from build123d import *

# Parameters (mm, degrees)
SKETCH1_R           = 2.032
BOSS_EXTRUDE1_DEPTH = 1.5875
FILLET1_R           = 6.35
FILLET2_R           = 3.175


with BuildPart() as part:
    # Sketch1 → Boss-Extrude1 (new body)
    with BuildSketch(Plane.XY):
        Polygon((9.525, -4.392368296), (9.525, 7.671504431), (3.175, 50.8), (-9.525, 50.8), (-15.875, 7.671504431), (-22.225, 1.957631704), (-22.225, -4.392368296), align=None)
        Circle(SKETCH1_R, mode=Mode.SUBTRACT)
        with Locations((-12.7, 0)):
            Circle(SKETCH1_R, mode=Mode.SUBTRACT)
    extrude(amount=BOSS_EXTRUDE1_DEPTH)

    # Fillet1
    fillet1_edges = [part.edges().sort_by_distance(p)[0] for p in [
        (-9.525, 50.8, 0.79375),
        (3.175, 50.8, 0.79375),
    ]]
    fillet(fillet1_edges, radius=FILLET1_R)

    # Fillet2
    fillet2_edges = [part.edges().sort_by_distance(p)[0] for p in [
        (-22.225, -4.392368296, 0.79375),
        (-22.225, 1.957631704, 0.79375),
        (-15.875, 7.671504431, 0.79375),
        (9.525, 7.671504431, 0.79375),
        (9.525, -4.392368296, 0.79375),
    ]]
    fillet(fillet2_edges, radius=FILLET2_R)


solid = part.part
Geometry check sheet. Reference: the model listing, model coordinates, mm. Round coordinates to 2 decimals unless told otherwise and drop trailing zeros. Order: outer loops, then holes, each group sorted by start corner. A loop starts at its lowest first (then second) coordinate and runs counter-clockwise, first axis right, second up. Notation, with made-up numbers: M 12.5,78 L 37.5,78 A21 ccw 37.5,98 Z; hole C 25.5,-21 d2. An arc over 180 degrees is marked long. Answer in a Markdown table with one row per item.
(1) Go/stop test with flat-tipped pins: P1, Ø6.5, axis at x = -12.7, y = 0, coming from the -Z side; P2, Ø1.5, axis at x = -16, y = 23, coming from the +Z side. Record where each tip stops, or that it passes through.
Responses:
| item | result |
|---|---|
| P1 | stops at z = 0 |
| P2 | passes through |
(2) Scan lines: probe 1 along Y at (x, z) = (0, 1.1); probe 2 along X at (y, z) = (19.5, 1.35); probe 3 along Y at (x, z) = (-5, 1.2). Record each from-to range of solid material in increasing order. Write a range as from..to.
Responses:
| item | result |
|---|---|
| probe 1 | y = -4.39..-2.03, 2.03..50.37 |
| probe 2 | x = -14.13..7.78 |
| probe 3 | y = -4.39..50.73 |
(3) Draft check along Y on faces 1 (the face through (-14.73, 0.09, 0.78)), 2 (the face through (-0.44, -1.984, 0.783)), 3 (the face through (-21.27, -3.49, 0.8)), 4 (the face through (-3, 50.8, 1)). Enter one of: released by +Y, released by -Y, zero draft, split by the parting line, or undercut.
Responses:
| item | result |
|---|---|
| face 1 | undercut |
| face 2 | undercut |
| face 3 | released by -Y |
| face 4 | released by +Y |
(4) Sectioned sample at D-D, the plane x = -12.7. Record the cut outline in (y, z).
Responses:
| item | result |
|---|---|
| outline | M -4.39,0 L -2.03,0 L -2.03,1.59 L -4.39,1.59 Z; M 2.03,0 L 29.24,0 L 29.24,1.59 L 2.03,1.59 Z |
(5) Sectioned sample at C-C, the plane x = -1. Record the cut outline in (y, z).
Responses:
| item | result |
|---|---|
| outline | M -4.39,0 L -1.77,0 L -1.77,1.59 L -4.39,1.59 Z; M 1.77,0 L 50.66,0 L 50.66,1.59 L 1.77,1.59 Z |
(6) Sectioned sample at B-B, the plane y = 0. Record the cut outline in (x, z) (1 decimal), and give its area (3 significant figures).
Responses:
| item | result |
|---|---|
| outline | M -22.2,0 L -14.7,0 L -14.7,1.6 L -22.2,1.6 Z; M -10.7,0 L -2,0 L -2,1.6 L -10.7,1.6 Z; M 2,0 L 9.5,0 L 9.5,1.6 L 2,1.6 Z |
| area | 37.5 mm² |
(7) Sectioned sample at A-A, the plane z = 0.6. State how many separate pieces and enclosed holes the cut face has, and give its area (3 significant figures).
Responses:
| item | result |
|---|---|
| separate pieces | 1 |
| enclosed holes | 2 |
| area | 1,140 mm² |
